Design review of the part built by this model. Coordinates are the model's own, in mm. A direction names the side the tool comes from. Give positions to 0.01 mm unless a question says otherwise; leave off trailing zeros. Loops run counter-clockwise (first coordinate to the right, second up) from the corner with the lowest first, then second, coordinate; pieces in that order, holes last. Notation, with made-up numbers: (60.5, 80.25) -> (77.5, 80.25) arc R11 cw to (77.5, 89.25) -> close; hole circle Ø2 at (-3.75, -31.5). An arc over 180 degrees is marked (long way). Answer as CSV lines item,"result".
from build123d import *

# Parameters (mm, degrees)
F0_W     = 190
F0_H     = 90
F0_W_2   = 10
F0_H_2   = 10
F0_R     = 4
F0_R_2   = 1.5
F1_DEPTH = 4
F2_DEPTH = 5
F3_DEPTH = 10


with BuildPart() as f1:
    # F0 (on Top) → F1 (new body)
    with BuildSketch(Plane.XY):
        Rectangle(F0_W, F0_H)
        with Locations((-85.5, -35.5)):
            Rectangle(F0_W_2, F0_H_2, mode=Mode.SUBTRACT)
        with Locations((-77.5, -20)):
            Circle(F0_R, mode=Mode.SUBTRACT)
        with Locations((85.5, -35.5)):
            Rectangle(F0_W_2, F0_H_2, mode=Mode.SUBTRACT)
        with Locations((77.5, -20)):
            Circle(F0_R, mode=Mode.SUBTRACT)
        with Locations((-85.5, 35.5)):
            Rectangle(F0_W_2, F0_H_2, mode=Mode.SUBTRACT)
        with Locations((85.5, 35.5)):
            Rectangle(F0_W_2, F0_H_2, mode=Mode.SUBTRACT)
        with Locations((-85.5, 35.5)):
            Rectangle(F0_W_2, F0_H_2)
        with Locations((-85.5, 35.5)):
            Circle(F0_R_2, mode=Mode.SUBTRACT)
        with Locations((77.5, -20)):
            Circle(F0_R)
        with Locations((77.5, -20)):
            Circle(F0_R_2, mode=Mode.SUBTRACT)
        with Locations((-77.5, -20)):
            Circle(F0_R)
        with Locations((-77.5, -20)):
            Circle(F0_R_2, mode=Mode.SUBTRACT)
        with Locations((85.5, -35.5)):
            Rectangle(F0_W_2, F0_H_2)
        with Locations((85.5, -35.5)):
            Circle(F0_R_2, mode=Mode.SUBTRACT)
        with Locations((-85.5, -35.5)):
            Rectangle(F0_W_2, F0_H_2)
        with Locations((-85.5, -35.5)):
            Circle(F0_R_2, mode=Mode.SUBTRACT)
        with Locations((85.5, 35.5)):
            Rectangle(F0_W_2, F0_H_2)
        with Locations((85.5, 35.5)):
            Circle(F0_R_2, mode=Mode.SUBTRACT)
        with Locations((85.5, -35.5)):
            Circle(F0_R_2)
        with Locations((-85.5, -35.5)):
            Circle(F0_R_2)
        with Locations((85.5, 35.5)):
            Circle(F0_R_2)
        with Locations((-85.5, 35.5)):
            Circle(F0_R_2)
        with Locations((77.5, -20)):
            Circle(F0_R_2)
        with Locations((-77.5, -20)):
            Circle(F0_R_2)
    extrude(amount=-F1_DEPTH)

    # F0 (on Top) → F2 (join)
    with BuildSketch(Plane.XY):
        with Locations((77.5, -20)):
            Circle(F0_R)
        with Locations((77.5, -20)):
            Circle(F0_R_2, mode=Mode.SUBTRACT)
        with Locations((-77.5, -20)):
            Circle(F0_R)
        with Locations((-77.5, -20)):
            Circle(F0_R_2, mode=Mode.SUBTRACT)
    extrude(amount=F2_DEPTH)

    # F0 (on Top) → F3 (join)
    with BuildSketch(Plane.XY):
        with Locations((-85.5, -35.5)):
            Rectangle(F0_W_2, F0_H_2)
        with Locations((-85.5, -35.5)):
            Circle(F0_R_2, mode=Mode.SUBTRACT)
        with Locations((-85.5, 35.5)):
            Rectangle(F0_W_2, F0_H_2)
        with Locations((-85.5, 35.5)):
            Circle(F0_R_2, mode=Mode.SUBTRACT)
        with Locations((85.5, 35.5)):
            Rectangle(F0_W_2, F0_H_2)
        with Locations((85.5, 35.5)):
            Circle(F0_R_2, mode=Mode.SUBTRACT)
        with Locations((85.5, -35.5)):
            Rectangle(F0_W_2, F0_H_2)
        with Locations((85.5, -35.5)):
            Circle(F0_R_2, mode=Mode.SUBTRACT)
    extrude(amount=F3_DEPTH)


solid = f1.part
Q1. The part is to be moulded in two halves that separate along X. For faces 1 (the cylindrical face through (74.55, -17.3, 2.46)), 2 (the flat face through (-1, -45, -2)), 3 (the flat face through (90.5, -36, 5)), say which applies: pulls with the +X half, pulls with the -X half, needs draft (parallel to the pull), parting line crosses it, or undercut.
Filled sheet:
face 1,"undercut"
face 2,"needs draft"
face 3,"pulls with the +X half"
Q2. Clearance check with flat-ended pins moving along their axes: pin 1 Ø3.5 at (x, y) = (77.5, -20) entering from +Z; pin 2 Ø8 at (x, z) = (-85, 5.5) entering from -Y; pin 3 Ø3 at (y, z) = (-35, 6) entering from -X. State where each tip first meets the part, or that it passes through.
Filled sheet:
pin 1,"stops at z = 5"
pin 2,"stops at y = -40.5"
pin 3,"stops at x = -90.5"
Q3. We need section B-B, the plane y = 2. State the section outline as (x, z) points.
Filled sheet:
outline,"(-95, -4) -> (95, -4) -> (95, 0) -> (-95, 0) -> close"
Q4. For faces 4 (the flat face through (-86, -30.5, 5)), 5 (the flat face through (80.5, -36, 5)), 6 (the flat face through (85, -40.5, 5)), 7 (the flat face through (80.5, 35, 5)), 8 (the flat face through (90.5, 35, 5)), list the 3-axis set-ups (+Z, -Z, +X, -X, +Y, -Y) from which the entire face can be reached by the end or side of a thin tool; tool diameter is ignored.
Filled sheet:
face 4,"+Z, +X, -X"
face 5,"+Z, -Y"
face 6,"+Z, +X, -X, -Y"
face 7,"+Z, +Y"
face 8,"+Z, +X, +Y, -Y"
Q5. We need section A-A, the plane x = -54.5. State the section outline as (y, z) points.
Filled sheet:
outline,"(-45, -4) -> (45, -4) -> (45, 0) -> (-45, 0) -> close"
Q6. To check wall thickness, follow probe 1 along Y at (x, z) = (85.5, 7.5); probe 2 along Y at (x, z) = (77.5, 1.1); probe 3 along Z at (x, y) = (68, 3). State the ranges of each line that lie inside material, in increasing order. Write a range as from..to.
Filled sheet:
probe 1,"y = -40.5..-37, -34..-30.5, 30.5..34, 37..40.5"
probe 2,"y = -24..-21.5, -18.5..-16"
probe 3,"z = -4..0"
